Could you check a few things on this model? Use its own coordinates, in mm. Face numbers are marked on the shaded views. Round coordinates to 2 decimals unless told otherwise and drop trailing zeros. Write each loop counter-clockwise with the first axis right and the second up, starting at its lowest first coordinate (ties: lowest second). Pieces come first, ordered by that corner, then holes. Notation, with made-up numbers: (-15, 75.25) -> (43, 75.25) arc R31 cw to (43, 113.25) -> close; hole circle Ø7 at (0, -14.5). An arc over 180 degrees is marked (long way). One line per question, with ' | ' between items. Start each with the question number.
1. Imagine slicing it at A-A, the plane y = 29.5. List the corners of the cut face in (x, z) for me (3 decimals).
2. For pin 1 Ø8 at (x, z) = (46.5, 10.5) entering from -Y; pin 2 Ø1.5 at (x, z) = (9, 29.5) entering from +Y; pin 3 Ø1 at (y, z) = (31.5, 5.5) entering from -X; pin 4 Ø4 at (x, y) = (4, 30) entering from -Z (3 decimals), each with a flat end and sliding along its axis, tell me the tip position at first contact or that it passes through.
3. Imagine slicing it at B-B, the plane z = 14. List the corners of the cut face in (x, y) for me (3 decimals), and give its area (3 significant figures).
4. Imagine slicing it at C-C, the plane x = -36. List the corners of the cut face in (y, z) for me (3 decimals).
5. Thinking about a two-plate mould opening in Z: for the marked faces 1 and 2, which applies, released by +Z, released by -Z, zero draft, split by the parting line, or undercut?
6. If I drill on line 1 along Z through (x, y) = (33, 33) (3 decimals); line 2 along X through (y, z) = (11.5, 7) (3 decimals); line 3 along Y through (x, z) = (-38.5, 16), over which ranges is the centre line in solid material (lowest first)? Write a range as [from, to].
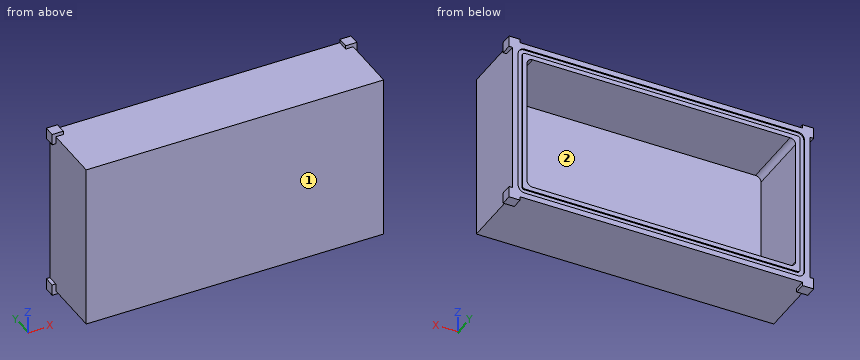
from build123d import *

# Parameters (mm, degrees)
SKETCH1_W           = 170.18
SKETCH1_H           = 95.25
BOSS_EXTRUDE1_DEPTH = 39.37
SKETCH2_W           = 153.67
SKETCH2_H           = 78.74
CUT_EXTRUDE1_DEPTH  = 37.592
SKETCH4_W           = 2.54
SKETCH4_H           = 1.524
FILLET1_R           = 3.175
SKETCH5_W           = 6.35
SKETCH5_H           = 6.35
BOSS_EXTRUDE2_DEPTH = 6.35


with BuildPart() as part:
    # Sketch1 → Boss-Extrude1 (new body)
    with BuildSketch(Plane(origin=(0, 0, 0), x_dir=(1, 0, 0), z_dir=(0, 1, 0))):
        Rectangle(SKETCH1_W, SKETCH1_H)
    extrude(amount=BOSS_EXTRUDE1_DEPTH)

    # Sketch2 → Cut-Extrude1 (cut)
    with BuildSketch(Plane(origin=(0, 39.37, 0), x_dir=(1, 0, 0), z_dir=(0, 1, 0))):
        Rectangle(SKETCH2_W, SKETCH2_H)
    extrude(amount=-CUT_EXTRUDE1_DEPTH, mode=Mode.SUBTRACT)

    # Cut-Sweep1: sweep along a path in Sketch3
    with BuildLine(Plane(origin=(0, 39.37, 0), x_dir=(1, 0, 0), z_dir=(0, 1, 0))) as cut_sweep1_path:
        Line((-78.105, -43.18), (78.105, -43.18))
        ThreePointArc((78.105, -43.18), (79.901051224, -42.436051224), (80.645, -40.64))
        Line((80.645, -40.64), (80.645, 40.64))
        ThreePointArc((80.645, 40.64), (79.901051224, 42.436051224), (78.105, 43.18))
        Line((78.105, 43.18), (-78.105, 43.18))
        ThreePointArc((-78.105, 43.18), (-79.901051224, 42.436051224), (-80.645, 40.64))
        Line((-80.645, 40.64), (-80.645, -40.64))
        ThreePointArc((-80.645, -40.64), (-79.901051224, -42.436051224), (-78.105, -43.18))
    # Sketch4 → Cut-Sweep1 (sweep, cut)
    with BuildSketch(Plane(origin=(-80.645, 39.37, 40.64), x_dir=(1, 0, 0), z_dir=(0, 0, 1))):
        Rectangle(SKETCH4_W, SKETCH4_H)
    sweep(path=cut_sweep1_path.line, mode=Mode.SUBTRACT)

    # Fillet1
    fillet1_edges = [part.edges().sort_by_distance(p)[0] for p in [
        (76.835, 20.574, 39.37),
        (-76.835, 20.574, 39.37),
        (-76.835, 20.574, -39.37),
        (76.835, 20.574, -39.37),
    ]]
    fillet(fillet1_edges, radius=FILLET1_R)

    # Sketch5 → Boss-Extrude2 (add)
    with BuildSketch(Plane(origin=(0, 39.37, 0), x_dir=(1, 0, 0), z_dir=(0, 1, 0))):
        with Locations((-83.974076836, 46.509076836)):
            Rectangle(SKETCH5_W, SKETCH5_H)
        with Locations((83.974076836, 46.509076836)):
            Rectangle(SKETCH5_W, SKETCH5_H)
        with Locations((83.974076836, -46.509076836)):
            Rectangle(SKETCH5_W, SKETCH5_H)
        with Locations((-83.974076836, -46.509076836)):
            Rectangle(SKETCH5_W, SKETCH5_H)
    extrude(amount=-BOSS_EXTRUDE2_DEPTH)


solid = part.part
Geometry results:
1) outline: (-85.09, -47.625) -> (85.09, -47.625) -> (85.09, 47.625) -> (-85.09, 47.625) -> close; hole (-76.835, -36.195) arc R3.175 ccw to (-73.66, -39.37) -> (73.66, -39.37) arc R3.175 ccw to (76.835, -36.195) -> (76.835, 36.195) arc R3.175 ccw to (73.66, 39.37) -> (-73.66, 39.37) arc R3.175 ccw to (-76.835, 36.195) -> close
2) pin 1: stops at y = 0 | pin 2: stops at y = 1.78 | pin 3: stops at x = -85.09 | pin 4: stops at z = -47.625
3) outline: (-85.09, 0) -> (85.09, 0) -> (85.09, 39.37) -> (81.915, 39.37) -> (81.915, 38.608) -> (79.375, 38.608) -> (79.375, 39.37) -> (76.835, 39.37) -> (76.835, 1.778) -> (-76.835, 1.778) -> (-76.835, 39.37) -> (-79.375, 39.37) -> (-79.375, 38.608) -> (-81.915, 38.608) -> (-81.915, 39.37) -> (-85.09, 39.37) -> close | area: 919 mm2
4) outline: (0, -47.625) -> (39.37, -47.625) -> (39.37, -44.45) -> (38.608, -44.45) -> (38.608, -41.91) -> (39.37, -41.91) -> (39.37, -39.37) -> (1.778, -39.37) -> (1.778, 39.37) -> (39.37, 39.37) -> (39.37, 41.91) -> (38.608, 41.91) -> (38.608, 44.45) -> (39.37, 44.45) -> (39.37, 47.625) -> (0, 47.625) -> close
5) face 1: zero draft | face 2: undercut
6) line 1: z = [-47.625, -39.37], [39.37, 47.625] | line 2: x = [-85.09, -76.835], [76.835, 85.09] | line 3: y = [0, 1.78]
